Can you work these out from the model? Positions are in its coordinate system, mm. Face numbers are marked on the shaded views. A direction names the side the tool comes from. Give positions to 0.01 mm unless a question says otherwise; leave off trailing zeros. Order: outer loops, then holes, each group sorted by start corner. A loop starts at its lowest first (then second) coordinate and runs counter-clockwise, first axis right, second up. Notation, with made-up numbers: (52, 3.25) - (75, 3.25) arc R16 ccw to (75, 19.25) - close; hole circle Ø6 at (-27.75, 87.5). An arc over 180 degrees is marked (long way). Answer as CSV lines item,"result".
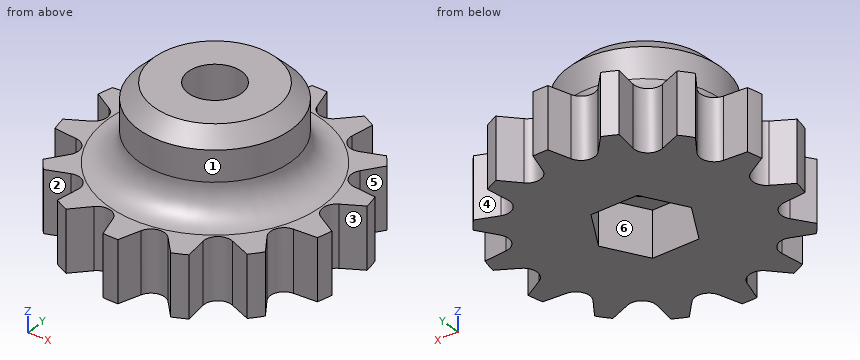
```python
from build123d import *

# Parameters (mm, degrees)
F2_R     = 1.75
F3_DEPTH = 12.5
F5_R     = 2
F7_DEPTH = 10
F8_R     = 1.75
F9_DEPTH = 3
F10_SIZE = 1


with BuildPart() as f1:
    # F0 (on Front) → F1 (revolve)
    with BuildSketch(Plane.XZ):
        Polygon((-9, -6), (0, -6), (0, 3), (-5, 3), (-5, -2), (-9, -2), align=None)
    revolve(axis=Axis((0, 0, -1.5), (0, 0, 1)))


with BuildPart() as f3:
    # F2 (on Top) → F3 (new body, symmetric)
    with BuildSketch(Plane.XY):
        Circle(F2_R)
    extrude(amount=F3_DEPTH, both=True)


with BuildPart() as f1_1:
    add(f1.part)

    # F4: cut F3
    add(f3.part, mode=Mode.SUBTRACT)

    # F5
    f5_edges = [f1_1.edges().sort_by_distance(p)[0] for p in [
        (5, 0, -2),
    ]]
    fillet(f5_edges, radius=F5_R)

    # F6 (on Top) → F7 (cut)
    with BuildSketch(Plane.XY):
        with BuildLine():
            ThreePointArc((-7.5796, -0.775802), (-7.13169, 0), (-7.5796, 0.775802))
            Line((-7.5796, 0.775802), (-10.312837, 2.353838))
            Line((-10.312837, 2.353838), (-10.499112, 2.339878))
            Line((-10.499112, 2.339878), (-10.499112, -2.339878))
            Line((-10.499112, -2.339878), (-10.312837, -2.353838))
            Line((-10.312837, -2.353838), (-7.5796, -0.775802))
        make_face()
        with BuildLine():
            Line((-10.474608, 2.447236), (-10.312837, 2.353838))
            Line((-10.312837, 2.353838), (-7.165591, 2.589691))
            ThreePointArc((-7.165591, 2.589691), (-6.425431, 3.094324), (-6.492375, 3.987639))
            Line((-6.492375, 3.987639), (-8.270253, 6.595307))
            Line((-8.270253, 6.595307), (-8.444138, 6.663552))
            Line((-8.444138, 6.663552), (-10.474608, 2.447236))
        make_face()
        Polygon((-10.499112, 2.396354), (-10.474608, 2.447236), (-10.499112, 2.461384), align=None)
        Polygon((-10.527328, 2.337764), (-10.499112, 2.339878), (-10.499112, 2.396354), align=None)
        with BuildLine():
            Line((-7.165591, -2.589691), (-10.312837, -2.353838))
            Line((-10.312837, -2.353838), (-10.474608, -2.447236))
            Line((-10.474608, -2.447236), (-8.444138, -6.663552))
            Line((-8.444138, -6.663552), (-8.270253, -6.595307))
            Line((-8.270253, -6.595307), (-6.492375, -3.987639))
            ThreePointArc((-6.492375, -3.987639), (-6.425431, -3.094324), (-7.165591, -2.589691))
        make_face()
        Polygon((-8.470477, 6.673889), (-8.444138, 6.663552), (-8.419634, 6.714434), align=None)
        Polygon((-10.499112, -2.396354), (-10.499112, -2.339878), (-10.527328, -2.337764), align=None)
        Polygon((-10.499112, -2.461384), (-10.474608, -2.447236), (-10.499112, -2.396354), align=None)
        with BuildLine():
            Line((-8.37548, 6.749646), (-8.270253, 6.595307))
            Line((-8.270253, 6.595307), (-5.33235, 5.442265))
            ThreePointArc((-5.33235, 5.442265), (-4.446536, 5.57578), (-4.119256, 6.409674))
            Line((-4.119256, 6.409674), (-4.589644, 9.530495))
            Line((-4.589644, 9.530495), (-4.716699, 9.667427))
            Line((-4.716699, 9.667427), (-8.37548, 6.749646))
        make_face()
        Polygon((-8.391419, 6.773024), (-8.419634, 6.714434), (-8.37548, 6.749646), align=None)
        Polygon((-8.419634, -6.714434), (-8.444138, -6.663552), (-8.470477, -6.673889), align=None)
        Polygon((-8.37548, -6.749646), (-8.419634, -6.714434), (-8.391419, -6.773024), align=None)
        with BuildLine():
            Line((-5.33235, -5.442265), (-8.270253, -6.595307))
            Line((-8.270253, -6.595307), (-8.37548, -6.749646))
            Line((-8.37548, -6.749646), (-4.716699, -9.667427))
            Line((-4.716699, -9.667427), (-4.589644, -9.530495))
            Line((-4.589644, -9.530495), (-4.119256, -6.409674))
            ThreePointArc((-4.119256, -6.409674), (-4.446536, -5.57578), (-5.33235, -5.442265))
        make_face()
        Polygon((-4.735944, 9.688168), (-4.716699, 9.667427), (-4.672544, 9.702639), align=None)
        with BuildLine():
            Line((-4.617485, 9.715206), (-4.589644, 9.530495))
            Line((-4.589644, 9.530495), (-2.442971, 7.216931))
            ThreePointArc((-2.442971, 7.216931), (-1.58695, 6.952884), (-0.930268, 7.562195))
            Line((-0.930268, 7.562195), (0, 10.578051))
            Line((0, 10.578051), (-0.055059, 10.756549))
            Line((-0.055059, 10.756549), (-4.617485, 9.715206))
        make_face()
        Polygon((-4.621702, 9.743184), (-4.672544, 9.702639), (-4.617485, 9.715206), align=None)
        Polygon((-4.672544, -9.702639), (-4.716699, -9.667427), (-4.735944, -9.688168), align=None)
        Polygon((-4.617485, -9.715206), (-4.672544, -9.702639), (-4.621702, -9.743184), align=None)
        with BuildLine():
            Line((-2.442971, -7.216931), (-4.589644, -9.530495))
            Line((-4.589644, -9.530495), (-4.617485, -9.715206))
            Line((-4.617485, -9.715206), (-0.055059, -10.756549))
            Line((-0.055059, -10.756549), (0, -10.578051))
            Line((0, -10.578051), (-0.930268, -7.562195))
            ThreePointArc((-0.930268, -7.562195), (-1.58695, -6.952884), (-2.442971, -7.216931))
        make_face()
        Polygon((-0.063399, 10.783587), (-0.055059, 10.756549), (0, 10.769116), align=None)
        with BuildLine():
            Line((0.055059, 10.756549), (0, 10.578051))
            Line((0, 10.578051), (0.930268, 7.562195))
            ThreePointArc((0.930268, 7.562195), (1.58695, 6.952884), (2.442971, 7.216931))
            Line((2.442971, 7.216931), (4.589644, 9.530495))
            Line((4.589644, 9.530495), (4.617485, 9.715206))
            Line((4.617485, 9.715206), (0.055059, 10.756549))
        make_face()
        Polygon((0.063399, 10.783587), (0, 10.769116), (0.055059, 10.756549), align=None)
        Polygon((0, -10.769116), (-0.055059, -10.756549), (-0.063399, -10.783587), align=None)
        Polygon((0.055059, -10.756549), (0, -10.769116), (0.063399, -10.783587), align=None)
        with BuildLine():
            Line((0.930268, -7.562195), (0, -10.578051))
            Line((0, -10.578051), (0.055059, -10.756549))
            Line((0.055059, -10.756549), (4.617485, -9.715206))
            Line((4.617485, -9.715206), (4.589644, -9.530495))
            Line((4.589644, -9.530495), (2.442971, -7.216931))
            ThreePointArc((2.442971, -7.216931), (1.58695, -6.952884), (0.930268, -7.562195))
        make_face()
        Polygon((4.621702, 9.743184), (4.617485, 9.715206), (4.672544, 9.702639), align=None)
        with BuildLine():
            Line((4.716699, 9.667427), (4.589644, 9.530495))
            Line((4.589644, 9.530495), (4.119256, 6.409674))
            ThreePointArc((4.119256, 6.409674), (4.446536, 5.57578), (5.33235, 5.442265))
            Line((5.33235, 5.442265), (8.270253, 6.595307))
            Line((8.270253, 6.595307), (8.37548, 6.749646))
            Line((8.37548, 6.749646), (4.716699, 9.667427))
        make_face()
        Polygon((4.735944, 9.688168), (4.672544, 9.702639), (4.716699, 9.667427), align=None)
        Polygon((4.672544, -9.702639), (4.617485, -9.715206), (4.621702, -9.743184), align=None)
        Polygon((4.716699, -9.667427), (4.672544, -9.702639), (4.735944, -9.688168), align=None)
        with BuildLine():
            Line((4.119256, -6.409674), (4.589644, -9.530495))
            Line((4.589644, -9.530495), (4.716699, -9.667427))
            Line((4.716699, -9.667427), (8.37548, -6.749646))
            Line((8.37548, -6.749646), (8.270253, -6.595307))
            Line((8.270253, -6.595307), (5.33235, -5.442265))
            ThreePointArc((5.33235, -5.442265), (4.446536, -5.57578), (4.119256, -6.409674))
        make_face()
        Polygon((8.391419, 6.773024), (8.37548, 6.749646), (8.419634, 6.714434), align=None)
        with BuildLine():
            Line((8.444138, 6.663552), (8.270253, 6.595307))
            Line((8.270253, 6.595307), (6.492375, 3.987639))
            ThreePointArc((6.492375, 3.987639), (6.425431, 3.094324), (7.165591, 2.589691))
            Line((7.165591, 2.589691), (10.312837, 2.353838))
            Line((10.312837, 2.353838), (10.474608, 2.447236))
            Line((10.474608, 2.447236), (8.444138, 6.663552))
        make_face()
        Polygon((8.470477, 6.673889), (8.419634, 6.714434), (8.444138, 6.663552), align=None)
        Polygon((8.419634, -6.714434), (8.37548, -6.749646), (8.391419, -6.773024), align=None)
        Polygon((8.444138, -6.663552), (8.419634, -6.714434), (8.470477, -6.673889), align=None)
        with BuildLine():
            Line((6.492375, -3.987639), (8.270253, -6.595307))
            Line((8.270253, -6.595307), (8.444138, -6.663552))
            Line((8.444138, -6.663552), (10.474608, -2.447236))
            Line((10.474608, -2.447236), (10.312837, -2.353838))
            Line((10.312837, -2.353838), (7.165591, -2.589691))
            ThreePointArc((7.165591, -2.589691), (6.425431, -3.094324), (6.492375, -3.987639))
        make_face()
        Polygon((10.499112, 2.461384), (10.474608, 2.447236), (10.499112, 2.396354), align=None)
        with BuildLine():
            Line((10.499112, 2.339878), (10.312837, 2.353838))
            Line((10.312837, 2.353838), (7.5796, 0.775802))
            ThreePointArc((7.5796, 0.775802), (7.13169, 0), (7.5796, -0.775802))
            Line((7.5796, -0.775802), (10.312837, -2.353838))
            Line((10.312837, -2.353838), (10.499112, -2.339878))
            Line((10.499112, -2.339878), (10.499112, 2.339878))
        make_face()
        Polygon((10.527328, 2.337764), (10.499112, 2.396354), (10.499112, 2.339878), align=None)
        Polygon((10.499112, -2.396354), (10.474608, -2.447236), (10.499112, -2.461384), align=None)
        Polygon((10.499112, -2.339878), (10.499112, -2.396354), (10.527328, -2.337764), align=None)
    extrude(amount=-F7_DEPTH, mode=Mode.SUBTRACT)

    # F8 (on face) → F9 (cut)
    with BuildSketch(Plane(origin=(0, 0, -6), x_dir=(1, 0, 0), z_dir=(0, 0, -1))):
        Polygon((-1.529978, -2.65), (1.529978, -2.65), (3.059956, 0), (1.529978, 2.65), (-1.529978, 2.65), (-3.059956, 0), align=None)
        Circle(F8_R, mode=Mode.SUBTRACT)
    extrude(amount=-F9_DEPTH, mode=Mode.SUBTRACT)

    # F10
    f10_edges = [f1_1.edges().sort_by_distance(p)[0] for p in [
        (5, 0, 3),
    ]]
    chamfer(f10_edges, length=F10_SIZE)


solid = f1_1.part
```
1) I'm going to push flat-ended pins straight in: P1, Ø4, axis at x = 1.5, z = -2.5, coming from the -Y side; P2, Ø4, axis at x = 0.5, y = 0, coming from the -Z side; P3, Ø1, axis at y = 4, z = 2, coming from the -X side. Where does each tip first touch, or does it pass through?
Answer block:
P1,"y = -9"
P2,"z = -3"
P3,"x = -3.57"
2) I want a section at B-B on z = 1.5. Write out the boundary of the cut face in (x, y).
Answer block:
outline,"circle Ø10 at (0, 0); hole circle Ø3.5 at (0, 0)"
3) Which directions (+Z, -Z, +X, -X, +Y, -Y) give clear straight access to the entire face, cutting with the end or side of a thin tool? Please do the marked faces 4, 5 and 6.
Answer block:
face 4,"+Z, -Z, +Y"
face 5,"+Z, -Z, +X"
face 6,"-Z"
4) I need wall thicknesses on line 1 along Y through (x, z) = (0, 0.5); line 2 along X through (y, z) = (-7.25, -2.75). Which ranges of each line are inside material? Lowest first, please. Write a range as [from, to].
Answer block:
line 1,"[-5, -1.75], [1.75, 5]"
line 2,"[-4.25, -2.47], [-1.1, 1.1], [2.47, 4.25]"
5) I want a section at A-A on x = 0. Write out the boundary of the cut face in (y, z).
Answer block:
outline,"(-9, -6) - (-2.65, -6) - (-2.65, -3) - (-1.75, -3) - (-1.75, 3) - (-4, 3) - (-5, 2) - (-5, 0) arc R2 cw to (-7, -2) - (-9, -2) - close; (1.75, -3) - (2.65, -3) - (2.65, -6) - (9, -6) - (9, -2) - (7, -2) arc R2 cw to (5, 0) - (5, 2) - (4, 3) - (1.75, 3) - close"
6) If we mould it in two halves opening along Y, with no side actions, what happens to the marked faces 1, 2 and 3? For each: +Y half, -Y half, draft (parallel to the pull), parting line (faces both ways), or undercut.
Answer block:
face 1,"parting line"
face 2,"-Y half"
face 3,"undercut"
7) I want a section at C-C on y = 5.75. Count the separate pieces of the cut face and the enclosed holes in it, plus the area to 3 significant figures.
Answer block:
separate pieces,"3"
enclosed holes,"0"
area,"42.5 mm2"
